Here's how the part is built. I have some questions about the finished solid (model axes, mm). A direction names the side the tool comes from. Give positions to 0.01 mm unless a question says otherwise; leave off trailing zeros. Loops run counter-clockwise (first coordinate to the right, second up) from the corner with the lowest first, then second, coordinate; pieces in that order, holes last. Notation, with made-up numbers: (-31, 15) - (15, 15) arc R12 ccw to (15, 25) - close; hole circle Ø5 at (21, 6.25). An arc over 180 degrees is marked (long way). Return JSON: item names as keys, results as strings. Group by question number.
(1) For P1, Ø4, axis at x = -4, y = 11, coming from the +Z side; P2, Ø1, axis at x = 12.5, z = 5.5, coming from the +Y side; P3, Ø2, axis at x = -12, z = 6, coming from the -Y side, each with a flat end and sliding along its axis, tell me the tip position at first contact or that it passes through.
(2) If we section it at A-A (z = 5.75): Please give me the cut outline in (x, y).
(3) On a 3-axis mill with a long thin cutter (end or side, diameter ignored), from which of +Z, -Z, +X, -X, +Y, -Y can I reach the whole of each face in a straight line? I mean faces 1 (the flat face through (8, 8, 6)), 2 (the flat face through (0, 12, 6)), 3 (the flat face through (5, -11, 4.5)), 4 (the flat face through (3.2, -8.1, 2)). Say none if no direction works.
(4) If we section it at B-B (z = 3.5): Please give me the cut outline in (x, y), then the cut area to 3 significant figures.
(5) If we mould it in two halves opening along Y, with no side actions, what happens to faces 5 (the flat face through (0, -12, 6)), 6 (the flat face through (-8, -8, 6)), 7 (the cylindrical face through (-3.47, 15.62, 0.49))? For each: released by +Y, released by -Y, zero draft, split by the parting line, or undercut.
(6) I need wall thicknesses on probe 1 along Y at (x, z) = (0, 0.65); probe 2 along Z at (x, y) = (-13, 4.5); probe 3 along Z at (x, y) = (-8.5, 9). Which ranges of each line are inside material? Lowest first, please. Write a range as [from, to].
Autodesk Inventor part; units mm, degrees
ref_plane "YZ Plane" through (0, 0, 0) normal (1, 0, 0) x (0, 1, 0)
ref_plane "XZ Plane" through (0, 0, 0) normal (0, 1, 0) x (-1, 0, 0)
ref_plane "XY Plane" through (0, 0, 0) normal (0, 0, 1) x (1, 0, 0)
sketch "Sketch1" plane through (0, 0, 0) normal (0, 0, 1) x (1, 0, 0)
  circle A0 centre (0, 0) radius 16
  circle A1 centre (0, 0) radius 8.5
  dimension "d0" = 32
  dimension "d1" = 17
extrude "Extrusion1" add sketch "Sketch1" along normal blind 2
sketch "Sketch2" plane through (0, 0, 2) normal (0, 0, 1) x (1, 0, 0)
  circle A0 centre (0, 0) radius 16
  circle A1 centre (0, 0) radius 11
  circle A2 centre (0, 0) radius 13
  dimension "d4" = 22
  dimension "d5" = 26
extrude "Extrusion2" add sketch "Sketch2" along normal blind 4.5 contours A2
sketch "Sketch3" plane through (0, 0, 6.5) normal (0, 0, 1) x (1, 0, 0)
  circle A0 centre (0, 0) radius 11
  circle A1 centre (0, 0) radius 13
  line L0 (-13, 0) -> (13, 0) construction
  line L1 (0, 13) -> (0, -13) construction
  line L2 (-9.1924, 9.1924) -> (9.1924, -9.1924) construction
  line L3 (9.1924, 9.1924) -> (-9.1924, -9.1924) construction
  circle A2 centre (0, 0) radius 13
  circle A3 centre (0, 0) radius 11
  line L4 (-13, 0) -> (-11, 0)
  line L5 (-7.7782, 7.7782) -> (-9.1924, 9.1924)
  line L6 (0, 13) -> (0, 11)
  line L7 (7.7782, 7.7782) -> (9.1924, 9.1924)
  line L8 (11, 0) -> (13, 0)
  line L9 (9.1924, -9.1924) -> (7.7782, -7.7782)
  line L10 (0, -11) -> (0, -13)
  line L11 (-7.7782, -7.7782) -> (-9.1924, -9.1924)
  dimension "d8" = 45
  dimension "d9" = 45
extrude "Extrusion3" cut sketch "Sketch3" against normal blind 2 contours A0 L7 A1 L8 | L9 A1 L10 A0 | A0 L5 A1 L6 | L11 A1 L4 A0
chamfer "Chamfer1" distance 1 angle 45 1 edges at (-16, 0, 2)
properties part number "belt_guide" material "ABS Plastic"
Values:
{
 "1": {"P1": "z = 4.5", "P2": "y = 0", "P3": "y = 0"},
 "2": {"outline": "(-13, 0) - (-11, 0) arc R11 cw to (-7.78, 7.78) - (-9.19, 9.19) arc R13 ccw to start; (-9.19, -9.19) arc R13 ccw to (0, -13) - (0, -11) arc R11 cw to (-7.78, -7.78) - close; (0, 11) arc R11 cw to (7.78, 7.78) - (9.19, 9.19) arc R13 ccw to (0, 13) - close; (7.78, -7.78) - (9.19, -9.19) arc R13 ccw to (13, 0) - (11, 0) arc R11 cw to start"},
 "3": {"face 1": "+Z, +X", "face 2": "+Z, -X, +Y", "face 3": "+Z, -Y", "face 4": "+Z"},
 "4": {"outline": "circle Ø26 at (0, 0); hole circle Ø22 at (0, 0)", "area": "151 mm2"},
 "5": {"face 5": "zero draft", "face 6": "undercut", "face 7": "split by the parting line"},
 "6": {"probe 1": "[-16, -8.5], [8.5, 16]", "probe 2": "[0, 2]", "probe 3": "[0, 4.5]"}
}
